Source: CAD feature listing. Evaluate the final solid. Frame: model axes, mm. Face numbers are marked on the shaded views. A direction names the side the tool comes from. Coordinates: 2 decimals unless noted, no trailing zeros. Order: outer loops, then holes, each group sorted by start corner. A loop starts at its lowest first (then second) coordinate and runs counter-clockwise, first axis right, second up.
```python
from build123d import *


with BuildPart() as part:
    # Sketch1 → Revolve1 (revolve)
    with BuildSketch(Plane.XY):
        with BuildLine():
            Line((0, -0.381), (0, -6.35))
            Line((0, -6.35), (0.5969, -6.35))
            ThreePointArc((0.5969, -6.35), (1.297359977, -6.059859977), (1.5875, -5.3594))
            Line((1.5875, -5.3594), (1.5875, -1.184098677))
            ThreePointArc((1.5875, -1.184098677), (1.611297822, -1.076753638), (1.678231947, -0.989523388))
            Line((1.678231947, -0.989523388), (2.706147294, -0.127))
            Line((2.706147294, -0.127), (2.706147294, 0))
            Line((2.706147294, 0), (0.381, 0))
            ThreePointArc((0.381, 0), (0.269407684, -0.269407684), (0, -0.381))
        make_face()
    revolve(axis=Axis((0, 28.449499207, 0), (0, -1, 0)))


solid = part.part
```
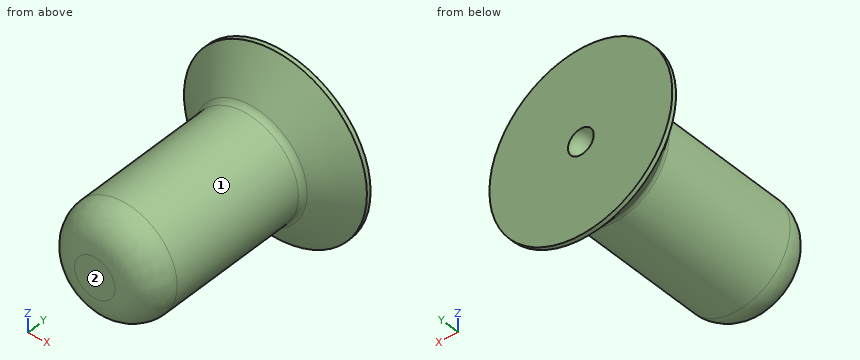
Q1. Set-up query: the marked faces 1 and 2. Return all of +Z, -Z, +X, -X, +Y, -Y with unobstructed straight access to the full face (end or side cutting, diameter ignored); none if empty.
Solutions:
face 1: -Y
face 2: +Z, -Z, +X, -X, -Y
Q2. Material intervals for line 1 along Y through (x, z) = (-1.8, 1.55); line 2 along X through (y, z) = (-0.5, -1.85); line 3 along Z through (x, y) = (0.1, -4), sorted ascending.
Solutions:
line 1: y = -0.4 to 0
line 2: x = -1.3 to 1.3
line 3: z = -1.58 to 1.58
Q3. Pin query (flat end, axial travel): P1, Ø3, axis at y = -2, z = 0, coming from the -X side; P2, Ø3, axis at y = -2, z = 1, coming from the -X side; P3, Ø1.5, axis at x = -1, y = -2, coming from the -Z side. Return the tip coordinate at first contact, or that it passes through.
Solutions:
P1: stops at x = -2.26
P2: stops at x = -2.11
P3: stops at z = -1.57
Q4. Section query A-A on y = -5. Output: boundary loops of the cut face in (x, z) (1 decimal), plus the area to 3 significant figures.
Solutions:
outline: circle Ø3.2 at (0, 0)
area: 7.92 mm2
